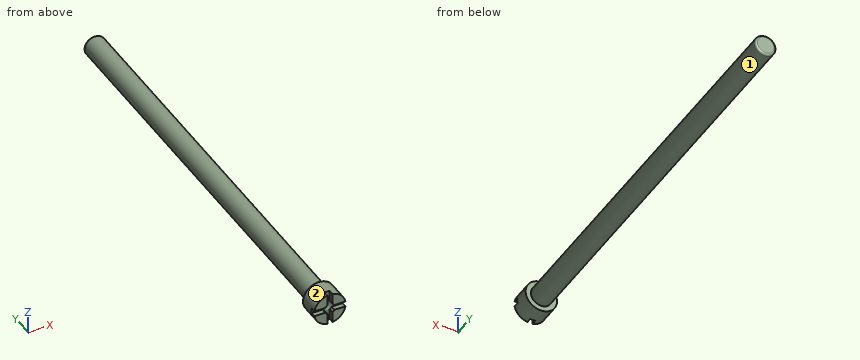
from build123d import *

# Parameters (mm, degrees)
SKETCH1_R           = 0.5
BOSS_EXTRUDE1_DEPTH = 20
SKETCH2_R           = 0.75
BOSS_EXTRUDE2_DEPTH = 1
CUT_EXTRUDE1_DEPTH  = 0.25
FILLET1_R           = 0.1


with BuildPart() as part:
    # Sketch1 → Boss-Extrude1 (new body)
    with BuildSketch(Plane(origin=(0, 0, 0), x_dir=(1, 0, 0), z_dir=(0, 1, 0))):
        with Locations(Location((0, 0, 0), (0, 0, 270))):
            Circle(SKETCH1_R)
    extrude(amount=BOSS_EXTRUDE1_DEPTH)

    # Sketch2 → Boss-Extrude2 (add)
    with BuildSketch(Plane.XZ):
        with Locations(Location((0, 0, 0), (0, 0, 270))):
            Circle(SKETCH2_R)
    extrude(amount=BOSS_EXTRUDE2_DEPTH)

    # Sketch3 → Cut-Extrude1 (cut)
    with BuildSketch(Plane.XZ.offset(1)):
        Polygon((-0.125, 0.125), (-0.875467833, 0.125), (-0.875467833, -0.125), (-0.125, -0.125), (-0.125, -0.835149175), (0.125, -0.835149175), (0.125, -0.125), (0.875467833, -0.125), (0.875467833, 0.125), (0.125, 0.125), (0.125, 0.835149175), (-0.125, 0.835149175), align=None)
    extrude(amount=-CUT_EXTRUDE1_DEPTH, mode=Mode.SUBTRACT)

    # Sketch5 → Cut-Revolve1 (revolve, cut)
    with BuildSketch(Plane(origin=(0, 0, 0), x_dir=(0, 0, -1), z_dir=(1, 0, 0)), mode=Mode.PRIVATE) as cut_revolve1_sk:
        Polygon((0, -0.659007441), (0, -1), (0.25, -1), (0.25, -0.75), align=None)
    revolve(cut_revolve1_sk.sketch.rotate(Axis((0, -0.659007441, 0), (0, 1, 0)), 170.405931773), axis=Axis((0, -0.659007441, 0), (0, 1, 0)), mode=Mode.SUBTRACT)

    # Fillet1
    fillet1_edges = [part.edges().sort_by_distance(p)[0] for p in [
        (0, 20, -0.5),
    ]]
    fillet(fillet1_edges, radius=FILLET1_R)


solid = part.part
Verification items for the finished model (mm, model axes). Face numbers are marked on the shaded views. A direction names the side the tool comes from. Give positions to 0.01 mm unless a question says otherwise; leave off trailing zeros. Write each loop counter-clockwise with the first axis right and the second up, starting at its lowest first coordinate (ties: lowest second). Pieces come first, ordered by that corner, then holes. Notation, with made-up numbers: M -37,19.25 L -28,19.25 A17 ccw -28,35.25 Z; hole C 81.5,49.5 d5. An arc over 180 degrees is marked long. Use CSV: the item, a comma, the result in double quotes.
1) Material ranges on line 1 along Y through (x, z) = (-0.55, 0.4); line 2 along X through (y, z) = (11, -0.3), recorded low to high.
Final values:
line 1,"-1 to 0"
line 2,"-0.4 to 0.4"
2) Access from +Z, -Z, +X, -X, +Y, -Y to the whole of each face (thin tool, end or side, straight path). Record for the marked faces 1 and 2.
Final values:
face 1,"+Y"
face 2,"+Y, -Y"
3) Cross-section at A-A (y = 13). Enter the section's corners in (x, z).
Final values:
outline,"C 0,0 d1"
